```python
from build123d import *

# Parameters (mm, degrees)
BOSS_EXTRUDE1_DEPTH = 30
TAP1_D              = 2.459
TAP1_DEPTH          = 8.5
TAP1_TIP            = 0.738758131


with BuildPart() as part:
    # Sketch1 → Boss-Extrude1 (new body)
    with BuildSketch(Plane(origin=(0, 0, 0), x_dir=(0, 0, -1), z_dir=(1, 0, 0))):
        Polygon((3, 1.732050808), (0, 3.464101615), (-3, 1.732050808), (-3, -1.732050808), (0, -3.464101615), (3, -1.732050808), align=None)
    extrude(amount=BOSS_EXTRUDE1_DEPTH)

    # Sketch2 → Cut-Revolve1 (revolve, cut)
    with BuildSketch(Plane.XY):
        Polygon((0, 3.464101615), (0.267949192, 3.464101615), (0, 3), align=None)
        Polygon((29.732050808, 3.464101615), (30, 3), (30, 3.464101615), align=None)
    revolve(axis=Axis((-88.99, 0, 0), (1, 0, 0)), mode=Mode.SUBTRACT)

    # Tap1
    with Locations(Plane(origin=(30, -0.086368032, -2.129727113), x_dir=(0, 0, -1), z_dir=(1, 0, 0))):
        with Locations((-2.129727113, 0.086368032)):
            Hole(TAP1_D / 2, depth=TAP1_DEPTH)
            with Locations((0, 0, -(TAP1_DEPTH + TAP1_TIP / 2))):  # 118° drill point
                Cone(0, TAP1_D / 2, TAP1_TIP, mode=Mode.SUBTRACT)

    # Sketch5 → Revolve1 (revolve)
    with BuildSketch(Plane.XY, mode=Mode.PRIVATE) as revolve1_sk:
        Polygon((0, 1.15), (-1, 1.15), (-1, 1.5), (-4.5, 1.5), (-4.5, 0), (0, 0), align=None)
    revolve(revolve1_sk.sketch.rotate(Axis((-88.99, 0, 0), (1, 0, 0)), 90), axis=Axis((-88.99, 0, 0), (1, 0, 0)))


solid = part.part
```
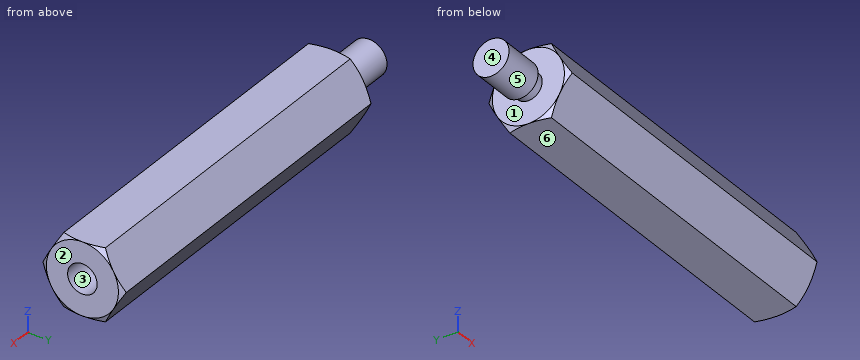
Geometry check sheet. Reference: the model listing, model coordinates, mm. Face numbers are marked on the shaded views. A direction names the side the tool comes from. Coordinates: 2 decimals unless noted, no trailing zeros. Order: outer loops, then holes, each group sorted by start corner. A loop starts at its lowest first (then second) coordinate and runs counter-clockwise, first axis right, second up.
Item 1: Tool access check on the marked faces 1 and 2. Record the directions out of +Z, -Z, +X, -X, +Y, -Y that give a thin tool (end or side, any length) a straight path to the whole face; none if there is none.
Item 2: Section check B-B (x = 18). Enter the section's corners in (y, z).
Item 3: Depth check by flat-ended pin: pin 1 (1.5 mm diameter, centred on y = 0, z = 0, fed in from +X); pin 2 (4 mm diameter, centred on x = 17.5, y = 2, fed in from +Z); pin 3 (1.5 mm diameter, centred on x = 8.5, z = -2.5, fed in from +Y). Enter the tip coordinate at first touch or a pass-through.
Item 4: Mould release check, pull along Z, two halves, no side actions. Record for the marked faces 3, 4, 5 and 6: released by +Z, released by -Z, zero draft, split by the parting line, or undercut.
Item 5: Scan lines: line 1 along Z through (x, y) = (27, 0); line 2 along X through (y, z) = (-0.25, -2.65); line 3 along Y through (x, z) = (23, 0.6). Record each from-to range of solid material in increasing order.
Item 6: Section check A-A (x = 24.5). Enter the section's corners in (y, z).
Check sheet entries:
1. face 1: none
1. face 2: +Z, -Z, +X, +Y, -Y
2. outline: (-3.46, 0) - (-1.73, -3) - (1.73, -3) - (3.46, 0) - (1.73, 3) - (-1.73, 3) - close
3. pin 1: stops at x = 21.21
3. pin 2: stops at z = 3
3. pin 3: stops at y = 2.45
4. face 3: undercut
4. face 4: zero draft
4. face 5: split by the parting line
4. face 6: released by -Z
5. line 1: z = -3 to -1.23, 1.23 to 3
5. line 2: x = 0 to 30
5. line 3: y = -3.12 to -1.07, 1.07 to 3.12
6. outline: (-3.46, 0) - (-1.73, -3) - (1.73, -3) - (3.46, 0) - (1.73, 3) - (-1.73, 3) - close; hole circle Ø2.46 at (0, 0)
